Check sheet for the modelled part. Datum: model origin and axes. Units: mm. A direction names the side the tool comes from. Give positions to 0.01 mm unless a question says otherwise; leave off trailing zeros. Write each loop counter-clockwise with the first axis right and the second up, starting at its lowest first coordinate (ties: lowest second). Pieces come first, ordered by that corner, then holes. Notation, with made-up numbers: M 7,80.25 L 57,80.25 A15 ccw 57,104.25 Z; hole C 41.5,31 d11. An arc over 180 degrees is marked long. Write item = value, one per line. Start each with the question number.
1) Set-up check for faces 5 (the face through (-2, 9, 5)), 6 (the face through (-0.4, 0.2, -385)): record each of +Z, -Z, +X, -X, +Y, -Y from which the full face is reachable in a straight line by a thin tool's end or side.
2) Scan lines: L1, parallel to Y at x = -19, z = -138; L2, parallel to X at y = 34, z = 133; L3, parallel to X at y = 39.4, z = -325. Record each from-to range of solid material in increasing order.
3) Draft check along X on faces 1 (the face through (-48.2, -33.7, 385)), 2 (the face through (-48, 28, 5)), 3 (the face through (0, -9, 5)), 4 (the face through (-50, -28, 5)). Enter one of: pulls with the +X half, pulls with the -X half, needs draft (parallel to the pull), parting line crosses it, or undercut.
4) Gauge pin test, flat ends, axial feed: pin 1 (1.6 mm diameter, centred on x = -1, z = 279.5, fed in from +Y); pin 2 (5 mm diameter, centred on y = -7.5, z = 7, fed in from -X); pin 3 (0.6 mm diameter, centred on x = -49, z = 75, fed in from -Y). Record the tip position at first contact, or that the pin passes through.
5) Sectioned sample at A-A, the plane z = -35. Record the cut outline in (x, y), then the cut area to 3 significant figures.
from build123d import *

# Parameters (mm, degrees)
SM_BASE_FLANGE_1_DEPTH = 385
CUT_EXTRUDE_1_DEPTH    = 10
CUT_EXTRUDE_2_DEPTH    = 10
SKETCH_8_R             = 2.5
CUT_EXTRUDE_3_DEPTH    = 10
CUT_EXTRUDE_START      = -10
CUT_EXTRUDE_4_DEPTH    = 10


# Sheet-metal steps are written as plain solids
with BuildPart() as part:
    # Sketch 1 → Базовая кромка1 (new, symmetric)
    with BuildSketch(Plane.XY):
        with BuildLine():
            Line((-50, -20), (-50, -36))
            ThreePointArc((-50, -36), (-48.828427125, -38.828427125), (-46, -40))
            Line((-46, -40), (-4, -40))
            ThreePointArc((-4, -40), (-1.171572875, -38.828427125), (0, -36))
            Line((0, -36), (0, 36))
            ThreePointArc((0, 36), (-1.171572875, 38.828427125), (-4, 40))
            Line((-4, 40), (-46, 40))
            ThreePointArc((-46, 40), (-48.828427125, 38.828427125), (-50, 36))
            Line((-50, 36), (-50, 20))
            Line((-50, 20), (-48, 20))
            Line((-48, 20), (-48, 36))
            ThreePointArc((-48, 36), (-47.414213562, 37.414213562), (-46, 38))
            Line((-46, 38), (-4, 38))
            ThreePointArc((-4, 38), (-2.585786438, 37.414213562), (-2, 36))
            Line((-2, 36), (-2, -36))
            ThreePointArc((-2, -36), (-2.585786438, -37.414213562), (-4, -38))
            Line((-4, -38), (-46, -38))
            ThreePointArc((-46, -38), (-47.414213562, -37.414213562), (-48, -36))
            Line((-48, -36), (-48, -20))
            Line((-48, -20), (-50, -20))
        make_face()
    extrude(amount=SM_BASE_FLANGE_1_DEPTH, both=True)

    # Эскиз6 → Вырез-Вытянуть1 (cut)
    with BuildSketch(Plane(origin=(0, 0, 0), x_dir=(0, 0, -1), z_dir=(1, 0, 0))):
        with BuildLine():
            Line((-364.5, 5.5), (-335.5, 5.5))
            ThreePointArc((-335.5, 5.5), (-330, 0), (-335.5, -5.5))
            Line((-335.5, -5.5), (-364.5, -5.5))
            ThreePointArc((-364.5, -5.5), (-370, 0), (-364.5, 5.5))
        make_face()
        with BuildLine():
            Line((-299.5, 5.5), (-270.5, 5.5))
            ThreePointArc((-270.5, 5.5), (-265, 0), (-270.5, -5.5))
            Line((-270.5, -5.5), (-299.5, -5.5))
            ThreePointArc((-299.5, -5.5), (-305, 0), (-299.5, 5.5))
        make_face()
        with BuildLine():
            Line((-234.5, 5.5), (-205.5, 5.5))
            ThreePointArc((-205.5, 5.5), (-200, 0), (-205.5, -5.5))
            Line((-205.5, -5.5), (-234.5, -5.5))
            ThreePointArc((-234.5, -5.5), (-240, 0), (-234.5, 5.5))
        make_face()
        with BuildLine():
            Line((-169.5, 5.5), (-140.5, 5.5))
            ThreePointArc((-140.5, 5.5), (-135, 0), (-140.5, -5.5))
            Line((-140.5, -5.5), (-169.5, -5.5))
            ThreePointArc((-169.5, -5.5), (-175, 0), (-169.5, 5.5))
        make_face()
        with BuildLine():
            Line((-104.5, 5.5), (-75.5, 5.5))
            ThreePointArc((-75.5, 5.5), (-70, 0), (-75.5, -5.5))
            Line((-75.5, -5.5), (-104.5, -5.5))
            ThreePointArc((-104.5, -5.5), (-110, 0), (-104.5, 5.5))
        make_face()
        with BuildLine():
            Line((-39.5, 5.5), (-10.5, 5.5))
            ThreePointArc((-10.5, 5.5), (-5, 0), (-10.5, -5.5))
            Line((-10.5, -5.5), (-39.5, -5.5))
            ThreePointArc((-39.5, -5.5), (-45, 0), (-39.5, 5.5))
        make_face()
        with BuildLine():
            Line((25.5, 5.5), (54.5, 5.5))
            ThreePointArc((54.5, 5.5), (60, 0), (54.5, -5.5))
            Line((54.5, -5.5), (25.5, -5.5))
            ThreePointArc((25.5, -5.5), (20, 0), (25.5, 5.5))
        make_face()
        with BuildLine():
            Line((90.5, 5.5), (119.5, 5.5))
            ThreePointArc((119.5, 5.5), (125, 0), (119.5, -5.5))
            Line((119.5, -5.5), (90.5, -5.5))
            ThreePointArc((90.5, -5.5), (85, 0), (90.5, 5.5))
        make_face()
        with BuildLine():
            Line((155.5, 5.5), (184.5, 5.5))
            ThreePointArc((184.5, 5.5), (190, 0), (184.5, -5.5))
            Line((184.5, -5.5), (155.5, -5.5))
            ThreePointArc((155.5, -5.5), (150, 0), (155.5, 5.5))
        make_face()
        with BuildLine():
            Line((220.5, 5.5), (249.5, 5.5))
            ThreePointArc((249.5, 5.5), (255, 0), (249.5, -5.5))
            Line((249.5, -5.5), (220.5, -5.5))
            ThreePointArc((220.5, -5.5), (215, 0), (220.5, 5.5))
        make_face()
        with BuildLine():
            Line((285.5, 5.5), (314.5, 5.5))
            ThreePointArc((314.5, 5.5), (320, 0), (314.5, -5.5))
            Line((314.5, -5.5), (285.5, -5.5))
            ThreePointArc((285.5, -5.5), (280, 0), (285.5, 5.5))
        make_face()
    extrude(amount=-CUT_EXTRUDE_1_DEPTH, mode=Mode.SUBTRACT)

    # Эскиз7 → Вырез-Вытянуть2 (cut)
    with BuildSketch(Plane(origin=(0, 40, 0), x_dir=(1, 0, 0), z_dir=(0, 1, 0))):
        with BuildLine():
            Line((-30.5, -385), (-30.5, -356))
            ThreePointArc((-30.5, -356), (-25, -350.5), (-19.5, -356))
            Line((-19.5, -356), (-19.5, -385))
            ThreePointArc((-19.5, -385), (-25, -390.5), (-30.5, -385))
        make_face()
        with BuildLine():
            Line((-31.5, -306), (-31.5, -259))
            ThreePointArc((-31.5, -259), (-25, -252.5), (-18.5, -259))
            Line((-18.5, -259), (-18.5, -306))
            ThreePointArc((-18.5, -306), (-25, -312.5), (-31.5, -306))
        make_face()
        with BuildLine():
            Line((-30.5, 385), (-30.5, 356))
            ThreePointArc((-30.5, 356), (-25, 350.5), (-19.5, 356))
            Line((-19.5, 356), (-19.5, 385))
            ThreePointArc((-19.5, 385), (-25, 390.5), (-30.5, 385))
        make_face()
        with BuildLine():
            Line((-31.5, 306), (-31.5, 259))
            ThreePointArc((-31.5, 259), (-25, 252.5), (-18.5, 259))
            Line((-18.5, 259), (-18.5, 306))
            ThreePointArc((-18.5, 306), (-25, 312.5), (-31.5, 306))
        make_face()
    extrude(amount=-CUT_EXTRUDE_2_DEPTH, mode=Mode.SUBTRACT)

    # Эскиз8 → Вырез-Вытянуть3 (cut)
    with BuildSketch(Plane(origin=(0, 40, 0), x_dir=(1, 0, 0), z_dir=(0, 1, 0))):
        with Locations(Location((-25, -325, 0), (0, 0, 270))):
            Circle(SKETCH_8_R)
        with Locations((-25, -275)):
            Circle(SKETCH_8_R)
        with Locations(Location((-25, -225, 0), (0, 0, 270))):
            Circle(SKETCH_8_R)
        with Locations(Location((-25, -175, 0), (0, 0, 270))):
            Circle(SKETCH_8_R)
        with Locations(Location((-25, -125, 0), (0, 0, 270))):
            Circle(SKETCH_8_R)
        with Locations(Location((-25, -75, 0), (0, 0, 270))):
            Circle(SKETCH_8_R)
        with Locations(Location((-25, -25, 0), (0, 0, 270))):
            Circle(SKETCH_8_R)
        with Locations(Location((-25, 25, 0), (0, 0, 270))):
            Circle(SKETCH_8_R)
        with Locations(Location((-25, 75, 0), (0, 0, 270))):
            Circle(SKETCH_8_R)
        with Locations(Location((-25, 125, 0), (0, 0, 270))):
            Circle(SKETCH_8_R)
        with Locations(Location((-25, 175, 0), (0, 0, 270))):
            Circle(SKETCH_8_R)
        with Locations(Location((-25, 225, 0), (0, 0, 270))):
            Circle(SKETCH_8_R)
        with Locations((-25, 275)):
            Circle(SKETCH_8_R)
        with Locations(Location((-25, 325, 0), (0, 0, 270))):
            Circle(SKETCH_8_R)
    extrude(amount=-CUT_EXTRUDE_3_DEPTH, mode=Mode.SUBTRACT)

    # Эскиз9 → Вырез-Вытянуть4 (cut)
    with BuildSketch(Plane.XZ.offset(40).offset(CUT_EXTRUDE_START)):
        with BuildLine():
            Line((-19.5, 385), (-19.5, 356))
            ThreePointArc((-19.5, 356), (-25, 350.5), (-30.5, 356))
            Line((-30.5, 356), (-30.5, 385))
            ThreePointArc((-30.5, 385), (-25, 390.5), (-19.5, 385))
        make_face()
        with BuildLine():
            Line((-30.5, -385), (-30.5, -356))
            ThreePointArc((-30.5, -356), (-25, -350.5), (-19.5, -356))
            Line((-19.5, -356), (-19.5, -385))
            ThreePointArc((-19.5, -385), (-25, -390.5), (-30.5, -385))
        make_face()
    extrude(amount=CUT_EXTRUDE_4_DEPTH, mode=Mode.SUBTRACT)


solid = part.part
Data:
q1.face_5 = +Z, -Z
q1.face_6 = -Z, +X, -X, +Y, -Y
q2.L1 = -40 to -38, 38 to 40
q2.L2 = -50 to -48, -2 to 0
q2.L3 = -48.11 to -27.5, -22.5 to -1.89
q3.face_1 = needs draft
q3.face_2 = undercut
q3.face_3 = pulls with the +X half
q3.face_4 = pulls with the -X half
q4.pin_1 = 39.34
q4.pin_2 = -2
q4.pin_3 = -38.95
q5.outline = M -50,-36 A4 ccw -46,-40 L -4,-40 A4 ccw 0,-36 L 0,-5.5 L -2,-5.5 L -2,-36 A2 cw -4,-38 L -46,-38 A2 cw -48,-36 L -48,-20 L -50,-20 Z; M -50,20 L -48,20 L -48,36 A2 cw -46,38 L -4,38 A2 cw -2,36 L -2,5.5 L 0,5.5 L 0,36 A4 ccw -4,40 L -46,40 A4 ccw -50,36 Z
q5.area = 392 mm2
